Check sheet for the modelled part. Datum: model origin and axes. Units: mm. Face numbers are marked on the shaded views. A direction names the side the tool comes from. Give positions to 0.01 mm unless a question says otherwise; leave off trailing zeros. Order: outer loops, then holes, each group sorted by start corner. A loop starts at its lowest first (then second) coordinate and runs counter-clockwise, first axis right, second up.
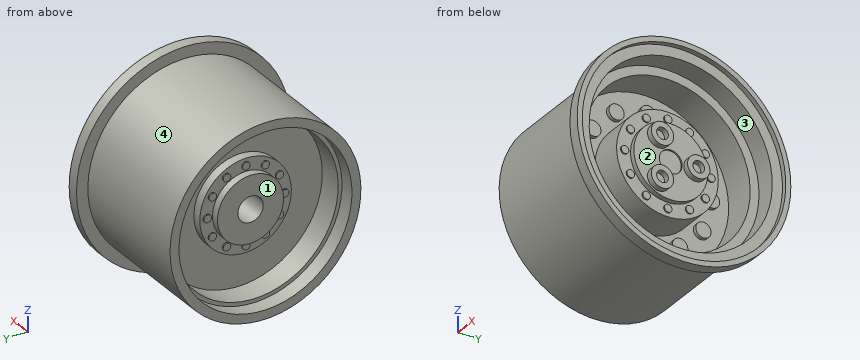
Solid Edge part; units mm, degrees
sketch "Sketch1" plane through (0, 0, 0) normal (0, -1, 0) x (1, 0, 0)
  line L0 (-2, -10.5) -> (-11.25, -10.5)
  line L1 (-11.25, -7.25) -> (-11.25, -10.5)
  line L2 (-10.5, -7.25) -> (-11.25, -7.25)
  line L3 (-10.5, -6) -> (-10.5, -7.25)
  line L4 (-9.6, -6) -> (-10.5, -6)
  line L5 (-9.6, -2.37) -> (-9.6, -6)
  line L6 (-12, -2.37) -> (-9.6, -2.37)
  line L7 (-12, -2) -> (-12, -2.37)
  line L8 (-13.5, -2) -> (-12, -2)
  line L9 (-13.5, -1.12) -> (-13.5, -2)
  line L10 (-1.1, -1.12) -> (-13.5, -1.12)
  line L11 (-1.1, 0) -> (-1.1, -1.12)
  line L12 (0, 0) -> (-1.1, 0)
  line L13 (0, 0) -> (0, -0.5)
  line L14 (0, -0.5) -> (-0.5, -0.5)
  line L15 (-0.5, -0.5) -> (-0.5, -1.5)
  line L16 (-0.5, -1.5) -> (-2.5, -1.5)
  line L17 (-2.5, -1.5) -> (-2.5, -2.37)
  line L18 (-2.5, -2.37) -> (-5.75, -2.37)
  line L19 (-5.75, -2.37) -> (-5.75, -5.5)
  line L20 (-5.75, -5.5) -> (-2.5, -5.5)
  line L21 (-2.5, -5.5) -> (-2.5, -6.87)
  line L22 (-2.5, -6.87) -> (-2, -6.87)
  line L23 (-2, -6.87) -> (-2, -10.5)
revolve "RevolvedProtrusion1" add sketch "Sketch1" angle 360 about axis through (-2, 0, -10.5) along (-1, 0, 0)
sketch "Sketch2" plane through (-5.75, 0, -10.5) normal (1, 0, 0) x (0, 0, -1)
  circle A0 centre (0, 6.25) radius 0.75
extrude "Protrusion1" add sketch "Sketch2" along normal mid plane 0.75
pattern_circular "Pattern1" count 12 over 360 about axis through (-5.75, 0, -10.5) along (-1, 0, 0) of "Protrusion1"
sketch "Sketch3" plane through (-2.5, 0, -10.5) normal (1, 0, 0) x (0, 0, -1)
  circle A0 centre (0, 4.25) radius 0.375
extrude "ExtrudedProtrusion_2" add sketch "Sketch3" along normal mid plane 0.25
pattern_circular "Pattern3" count 12 over 360 about axis through (-2.5, 0, -10.5) along (-1, 0, 0) of "ExtrudedProtrusion_2"
sketch "Sketch4" plane through (-2, 0, -10.5) normal (1, 0, 0) x (0, 0, -1)
  circle A0 centre (0, 0) radius 1.125
extrude "ExtrudedCutout_1" cut sketch "Sketch4" against normal blind 0.15
sketch "Sketch5" plane through (-2, 0, -10.5) normal (1, 0, 0) x (0, 0, -1)
  circle A0 centre (0, 2.375) radius 1.1
  circle A1 centre (0, 2.375) radius 0.575
extrude "ExtrudedProtrusion_3" add sketch "Sketch5" along normal mid plane 1.15
pattern_circular "Pattern5" count 3 over 360 about axis through (-1.425, 0, -10.5) along (-1, 0, 0) of "ExtrudedProtrusion_3"
sketch "Sketch6" plane through (-10.5, 0, -10.5) normal (-1, 0, 0) x (0, 0, 1)
  circle A0 centre (0, 3.81) radius 0.375
extrude "ExtrudedProtrusion_4" add sketch "Sketch6" along normal mid plane 0.25
pattern_circular "Pattern7" count 12 over 360 about axis through (-10.5, 0, -10.5) along (1, 0, 0) of "ExtrudedProtrusion_4"
sketch "Sketch7" plane through (-11.25, 0, -10.5) normal (-1, 0, 0) x (0, 0, 1)
  circle A0 centre (0, 0) radius 1.25
extrude "ExtrudedCutout_2" cut sketch "Sketch7" against normal blind 5
properties material "Stainless Steel, 420"
Q1. Tool access check on the marked faces 1 and 2. Record the directions out of +Z, -Z, +X, -X, +Y, -Y that give a thin tool (end or side, any length) a straight path to the whole face; none if there is none.
Q2. Sectioned sample at A-A, the plane x = -4.5. Record the cut outline in (y, z), plus the area to 3 significant figures.
Q3. Material ranges on line 1 (Y direction, x = -4.8, z = -10.5); line 2 (X direction, y = 3.75, z = -1.5); line 3 (Y direction, x = -1.25, z = -10.5), recorded low to high.
Q4. Sectioned sample at B-B, the plane z = -18.25. Record the cut outline in (x, y).
Q5. Sectioned sample at C-C, the plane x = -9.25. Record the cut outline in (y, z), plus the area to 3 significant figures.
Q6. Draft check along Z on the marked faces 3 and 4. Enter one of: pulls with the +Z half, pulls with the -Z half, needs draft (parallel to the pull), parting line crosses it, or undercut.
Q7. Go/stop test with flat-tipped pins: P1, Ø1, axis at x = -5, z = -9.5, coming from the +Y side; P2, Ø6, axis at x = -6, y = 3.5, coming from the -Z side; P3, Ø0.8, axis at y = -3, z = -12.5, coming from the -X side. Record where each tip stops, or that it passes through.
Filled in:
1. face 1: -X
1. face 2: +X
2. outline: circle Ø18.76 at (0, -10.5); circle Ø10 at (0, -10.5); hole circle Ø16.26 at (0, -10.5)
2. area: 147 mm2
3. line 1: y = -9.38 to -8.13, -5 to 5, 8.13 to 9.38
3. line 2: x = -1.1 to -0.5
3. line 3: y = -9.38 to -9, 9 to 9.38
4. outline: (-13.5, -5.28) - (-1.1, -5.28) - (-1.1, -7.08) - (0, -7.08) - (0, -6.32) - (-0.5, -6.32) - (-0.5, -4.58) - (-2.5, -4.58) - (-2.5, -2.46) - (-5.75, -2.46) - (-5.75, 2.46) - (-2.5, 2.46) - (-2.5, 4.58) - (-0.5, 4.58) - (-0.5, 6.32) - (0, 6.32) - (0, 7.08) - (-1.1, 7.08) - (-1.1, 5.28) - (-13.5, 5.28) - (-13.5, 3.49) - (-12, 3.49) - (-12, 2.46) - (-9.6, 2.46) - (-9.6, -2.46) - (-12, -2.46) - (-12, -3.49) - (-13.5, -3.49) - close
5. outline: circle Ø18.76 at (0, -10.5); hole circle Ø2.5 at (0, -10.5)
5. area: 272 mm2
6. face 3: undercut
6. face 4: parting line crosses it
7. P1: stops at y = 9.37
7. P2: stops at z = -19.87
7. P3: stops at x = -11.25
